Model file for the job. Use its own axes, mm. A direction names the side the tool comes from. Coordinates: 2 decimals unless noted, no trailing zeros. Order: outer loops, then holes, each group sorted by start corner. A loop starts at its lowest first (then second) coordinate and runs counter-clockwise, first axis right, second up. Notation, with made-up numbers: (-3, 29) -> (23, 29) arc R24 cw to (23, 54) -> close; hole circle Ø4 at (-3, 10). An arc over 180 degrees is marked (long way). Return JSON: item names as keys, results as strings. Group by question number.
1) Pull direction Y, two halves, no side cores. Call faces 1 (the flat face through (13, -4, -166.967)), 2 (the flat face through (25.4, 1, -84)), 3 (the flat face through (13, 17.198, -81)): +Y half, -Y half, draft (parallel to the pull), parting line (faces both ways), or undercut.
2) Cut at B-B (z = -77). Write the cut outline in (x, y), and give its area (3 significant figures).
3) Probe line 1 (Z direction, x = 15.25, y = 1.5); line 2 (Z direction, x = 1, y = -6); line 3 (Z direction, x = 2.75, y = -29.5). List the from-to ranges inside material, lowest first.
4) Which spindle directions (+Z, -Z, +X, -X, +Y, -Y) get a long thin tool onto all of the face, cutting with end or side? Do faces 4 (the cylindrical face through (22.9, -9.76, 2.17)), 5 (the flat face through (13, 20.574, -177)), 6 (the flat face through (0, 1, -84)), 7 (the flat face through (13, -17.198, -83)), 8 (the flat face through (4, -26.924, -177)). Say none if no direction does.
5) Cut at A-A (x = 12). State how many separate pieces and enclosed holes the cut face has, and give its area (3 significant figures).
6) Flat gauge pins, fed straight in: pin 1 (4 mm diameter, centred on x = 9.5, y = 14.5, fed in from +Z); pin 2 (2.5 mm diameter, centred on y = 1.56, z = -7.45, fed in from -X); pin 3 (10 mm diameter, centred on y = 0.5, z = 1.5, fed in from +X); pin 4 (4 mm diameter, centred on x = 6, y = 4, fed in from -Z). Where does each tip first touch, or does it go through?
from build123d import *

# Parameters (mm, degrees)
BOSS_EXTRUDE1_DEPTH = 25.4
FILLET1_R           = 2.54
SKETCH2_R           = 10
CUT_EXTRUDE2_DEPTH  = 5.08
CUT_EXTRUDE3_REACH  = 209.515
SKETCH6_W           = 20.066
SKETCH6_H           = 41.148
SKETCH9_W           = 20.066
SKETCH9_H           = 6.35
CUT_EXTRUDE6_DEPTH  = 7.62
FILLET2_R           = 1.27
CUT_EXTRUDE7_REACH  = 209.515
SKETCH10_R          = 0.75


with BuildPart() as part:
    # Sketch1 → Boss-Extrude1 (new body)
    with BuildSketch(Plane(origin=(0, 0, 0), x_dir=(0, 0, -1), z_dir=(1, 0, 0))):
        with BuildLine():
            Line((33.997808163, 17.197646354), (130.301908565, 17.197646354))
            ThreePointArc((130.301908565, 17.197646354), (202.399716728, 0), (130.301908565, -17.197646354))
            Line((130.301908565, -17.197646354), (33.997808163, -17.197646354))
            ThreePointArc((33.997808163, -17.197646354), (-38.1, 0), (33.997808163, 17.197646354))
        make_face()
    extrude(amount=BOSS_EXTRUDE1_DEPTH)

    # Fillet1
    fillet1_edges = [part.edges().sort_by_distance(p)[0] for p in [
        (12.7, 17.197646354, -33.997808163),
        (12.7, 17.197646354, -130.301908565),
        (12.7, -17.197646354, -130.301908565),
        (12.7, -17.197646354, -33.997808163),
    ]]
    fillet(fillet1_edges, radius=FILLET1_R)

    # Sketch2 → Cut-Extrude2 (cut)
    with BuildSketch(Plane(origin=(25.4, 0, 0), x_dir=(0, 0, -1), z_dir=(1, 0, 0))):
        Circle(SKETCH2_R)
    extrude(amount=-CUT_EXTRUDE2_DEPTH, mode=Mode.SUBTRACT)

    # Sketch6 → Cut-Extrude3 (cut, up to next)
    with BuildSketch(Plane(origin=(25.4, 0, 0), x_dir=(0, 0, -1), z_dir=(1, 0, 0)), mode=Mode.PRIVATE) as cut_extrude3_sk1:
        with Locations((176.999716728, 0)):
            Rectangle(SKETCH6_W, SKETCH6_H)
    cut_extrude3_tool1 = extrude(cut_extrude3_sk1.sketch, amount=-CUT_EXTRUDE3_REACH, mode=Mode.PRIVATE) & part.part
    add(cut_extrude3_tool1.solids().sort_by_distance((25.4, 0, -176.999717))[0], mode=Mode.SUBTRACT)

    # Sketch9 → Cut-Extrude6 (cut)
    with BuildSketch(Plane.ZY):
        with Locations((-176.999716728, -23.749)):
            Rectangle(SKETCH9_W, SKETCH9_H)
    extrude(amount=-CUT_EXTRUDE6_DEPTH, mode=Mode.SUBTRACT)

    # Fillet2
    fillet2_edges = [part.edges().sort_by_distance(p)[0] for p in [
        (7.62, -26.924, -176.999716728),
        (0, -26.924, -176.999716728),
    ]]
    fillet(fillet2_edges, radius=FILLET2_R)

    # Sketch10 → Cut-Extrude7 (cut, up to next)
    with BuildSketch(Plane.ZY, mode=Mode.PRIVATE) as cut_extrude7_sk1:
        with Locations((-4.019820442, -5.730710568)):
            Circle(SKETCH10_R)
    cut_extrude7_tool1 = extrude(cut_extrude7_sk1.sketch, amount=-CUT_EXTRUDE7_REACH, mode=Mode.PRIVATE) & part.part
    # Sketch10 → Cut-Extrude7 (cut, up to next)
    with BuildSketch(Plane.ZY, mode=Mode.PRIVATE) as cut_extrude7_sk2:
        with Locations((-6.475839257, -4.007930379)):
            Circle(SKETCH10_R)
    cut_extrude7_tool2 = extrude(cut_extrude7_sk2.sketch, amount=-CUT_EXTRUDE7_REACH, mode=Mode.PRIVATE) & part.part
    # Sketch10 → Cut-Extrude7 (cut, up to next)
    with BuildSketch(Plane.ZY, mode=Mode.PRIVATE) as cut_extrude7_sk3:
        with Locations((-1.563801627, -7.453490757)):
            Circle(SKETCH10_R)
    cut_extrude7_tool3 = extrude(cut_extrude7_sk3.sketch, amount=-CUT_EXTRUDE7_REACH, mode=Mode.PRIVATE) & part.part
    # Sketch10 → Cut-Extrude7 (cut, up to next)
    with BuildSketch(Plane.ZY, mode=Mode.PRIVATE) as cut_extrude7_sk4:
        with Locations((4.007930379, -6.475839257)):
            Circle(SKETCH10_R)
    cut_extrude7_tool4 = extrude(cut_extrude7_sk4.sketch, amount=-CUT_EXTRUDE7_REACH, mode=Mode.PRIVATE) & part.part
    # Sketch10 → Cut-Extrude7 (cut, up to next)
    with BuildSketch(Plane.ZY, mode=Mode.PRIVATE) as cut_extrude7_sk5:
        with Locations((5.730710568, -4.019820442)):
            Circle(SKETCH10_R)
    cut_extrude7_tool5 = extrude(cut_extrude7_sk5.sketch, amount=-CUT_EXTRUDE7_REACH, mode=Mode.PRIVATE) & part.part
    # Sketch10 → Cut-Extrude7 (cut, up to next)
    with BuildSketch(Plane.ZY, mode=Mode.PRIVATE) as cut_extrude7_sk6:
        with Locations((7.453490757, -1.563801627)):
            Circle(SKETCH10_R)
    cut_extrude7_tool6 = extrude(cut_extrude7_sk6.sketch, amount=-CUT_EXTRUDE7_REACH, mode=Mode.PRIVATE) & part.part
    # Sketch10 → Cut-Extrude7 (cut, up to next)
    with BuildSketch(Plane.ZY, mode=Mode.PRIVATE) as cut_extrude7_sk7:
        with Locations((6.475839257, 4.007930379)):
            Circle(SKETCH10_R)
    cut_extrude7_tool7 = extrude(cut_extrude7_sk7.sketch, amount=-CUT_EXTRUDE7_REACH, mode=Mode.PRIVATE) & part.part
    # Sketch10 → Cut-Extrude7 (cut, up to next)
    with BuildSketch(Plane.ZY, mode=Mode.PRIVATE) as cut_extrude7_sk8:
        with Locations((4.019820442, 5.730710568)):
            Circle(SKETCH10_R)
    cut_extrude7_tool8 = extrude(cut_extrude7_sk8.sketch, amount=-CUT_EXTRUDE7_REACH, mode=Mode.PRIVATE) & part.part
    # Sketch10 → Cut-Extrude7 (cut, up to next)
    with BuildSketch(Plane.ZY, mode=Mode.PRIVATE) as cut_extrude7_sk9:
        with Locations((1.563801627, 7.453490757)):
            Circle(SKETCH10_R)
    cut_extrude7_tool9 = extrude(cut_extrude7_sk9.sketch, amount=-CUT_EXTRUDE7_REACH, mode=Mode.PRIVATE) & part.part
    # Sketch10 → Cut-Extrude7 (cut, up to next)
    with BuildSketch(Plane.ZY, mode=Mode.PRIVATE) as cut_extrude7_sk10:
        with Locations((-4.007930379, 6.475839257)):
            Circle(SKETCH10_R)
    cut_extrude7_tool10 = extrude(cut_extrude7_sk10.sketch, amount=-CUT_EXTRUDE7_REACH, mode=Mode.PRIVATE) & part.part
    # Sketch10 → Cut-Extrude7 (cut, up to next)
    with BuildSketch(Plane.ZY, mode=Mode.PRIVATE) as cut_extrude7_sk11:
        with Locations((-5.730710568, 4.019820442)):
            Circle(SKETCH10_R)
    cut_extrude7_tool11 = extrude(cut_extrude7_sk11.sketch, amount=-CUT_EXTRUDE7_REACH, mode=Mode.PRIVATE) & part.part
    # Sketch10 → Cut-Extrude7 (cut, up to next)
    with BuildSketch(Plane.ZY, mode=Mode.PRIVATE) as cut_extrude7_sk12:
        with Locations((-7.453490757, 1.563801627)):
            Circle(SKETCH10_R)
    cut_extrude7_tool12 = extrude(cut_extrude7_sk12.sketch, amount=-CUT_EXTRUDE7_REACH, mode=Mode.PRIVATE) & part.part
    add(cut_extrude7_tool1.solids().sort_by_distance((0, -5.730711, -4.01982))[0], mode=Mode.SUBTRACT)
    add(cut_extrude7_tool2.solids().sort_by_distance((0, -4.00793, -6.475839))[0], mode=Mode.SUBTRACT)
    add(cut_extrude7_tool3.solids().sort_by_distance((0, -7.453491, -1.563802))[0], mode=Mode.SUBTRACT)
    add(cut_extrude7_tool4.solids().sort_by_distance((0, -6.475839, 4.00793))[0], mode=Mode.SUBTRACT)
    add(cut_extrude7_tool5.solids().sort_by_distance((0, -4.01982, 5.730711))[0], mode=Mode.SUBTRACT)
    add(cut_extrude7_tool6.solids().sort_by_distance((0, -1.563802, 7.453491))[0], mode=Mode.SUBTRACT)
    add(cut_extrude7_tool7.solids().sort_by_distance((0, 4.00793, 6.475839))[0], mode=Mode.SUBTRACT)
    add(cut_extrude7_tool8.solids().sort_by_distance((0, 5.730711, 4.01982))[0], mode=Mode.SUBTRACT)
    add(cut_extrude7_tool9.solids().sort_by_distance((0, 7.453491, 1.563802))[0], mode=Mode.SUBTRACT)
    add(cut_extrude7_tool10.solids().sort_by_distance((0, 6.475839, -4.00793))[0], mode=Mode.SUBTRACT)
    add(cut_extrude7_tool11.solids().sort_by_distance((0, 4.01982, -5.730711))[0], mode=Mode.SUBTRACT)
    add(cut_extrude7_tool12.solids().sort_by_distance((0, 1.563802, -7.453491))[0], mode=Mode.SUBTRACT)


solid = part.part
Answers below:
{
 "1": {"face 1": "undercut", "face 2": "draft", "face 3": "+Y half"},
 "2": {"outline": "(0, -17.2) -> (25.4, -17.2) -> (25.4, 17.2) -> (0, 17.2) -> close", "area": "874 mm^2"},
 "3": {"line 1": "z = -202.37 to -187.03, -166.97 to -8.2, -6.71 to 38.07", "line 2": "z = -201.92 to -187.03, -166.97 to -4.72, -3.32 to 3.43, 4.59 to 37.62", "line 3": "z = -188.41 to -140.19, -24.11 to 24.11"},
 "4": {"face 4": "+X", "face 5": "+X, -X", "face 6": "+Z, -Z, -X, +Y, -Y", "face 7": "+X, -X, -Y", "face 8": "-X"},
 "5": {"separate pieces": "1", "enclosed holes": "13", "area": "11,400 mm^2"},
 "6": {"pin 1": "stops at z = 35.99", "pin 2": "stops at x = 0", "pin 3": "stops at x = 20.32", "pin 4": "stops at z = -202.35"}
}
